Read the model definition and answer for the solid it produces. Units are mm, in the model's axes. Face numbers are marked on the shaded views. A direction names the side the tool comes from. Give positions to 0.01 mm unless a question says otherwise; leave off trailing zeros. Write each loop counter-clockwise with the first axis right and the second up, starting at its lowest first coordinate (ties: lowest second). Pieces come first, ordered by that corner, then holes. Notation, with made-up numbers: M -25,-20.5 L -7,-20.5 A32 cw -7,11.5 Z; hole C 87.5,0 d2. An arc over 180 degrees is marked long. Put each result on its own line as item: value.
from build123d import *

# Parameters (mm, degrees)
SKETCH1_W           = 84.03
SKETCH1_H           = 44.97
SKETCH1_W_2         = 0.71
SKETCH1_H_2         = 0.71
BOSS_EXTRUDE1_DEPTH = 4.61
CUT_EXTRUDE1_REACH  = 6.61
SKETCH2_R           = 1.25
SKETCH2_3_W         = 7.27
SKETCH2_3_H         = 4.6
CUT_EXTRUDE2_DEPTH  = 2.45
SKETCH2_4_R         = 6.72
SKETCH2_4_R_2       = 5.64
CUT_EXTRUDE3_DEPTH  = 1.75
SKETCH2_5_W         = 5.16
SKETCH2_5_H         = 14.14
SKETCH2_5_W_2       = 4.69
SKETCH2_5_H_2       = 2.4
SKETCH2_5_W_3       = 6.54
SKETCH2_5_H_3       = 7.3
SKETCH2_5_W_4       = 2.72
SKETCH2_5_H_4       = 6.27
CUT_EXTRUDE4_DEPTH  = 0.75


with BuildPart() as part:
    # Sketch1 → Boss-Extrude1 (new body)
    with BuildSketch(Plane(origin=(0, 0, 0), x_dir=(1, 0, 0), z_dir=(0, 1, 0))):
        with Locations((-42.015, -22.485)):
            Rectangle(SKETCH1_W, SKETCH1_H)
        with Locations((-74.615, -42.285)):
            Rectangle(SKETCH1_W_2, SKETCH1_H_2, mode=Mode.SUBTRACT)
        with Locations((-72.075, -42.285)):
            Rectangle(SKETCH1_W_2, SKETCH1_H_2, mode=Mode.SUBTRACT)
        with Locations((-69.535, -42.285)):
            Rectangle(SKETCH1_W_2, SKETCH1_H_2, mode=Mode.SUBTRACT)
        with Locations((-66.995, -42.285)):
            Rectangle(SKETCH1_W_2, SKETCH1_H_2, mode=Mode.SUBTRACT)
        with Locations((-64.455, -42.285)):
            Rectangle(SKETCH1_W_2, SKETCH1_H_2, mode=Mode.SUBTRACT)
        with Locations((-61.915, -42.285)):
            Rectangle(SKETCH1_W_2, SKETCH1_H_2, mode=Mode.SUBTRACT)
        with Locations((-59.375, -42.285)):
            Rectangle(SKETCH1_W_2, SKETCH1_H_2, mode=Mode.SUBTRACT)
        with Locations((-56.835, -42.285)):
            Rectangle(SKETCH1_W_2, SKETCH1_H_2, mode=Mode.SUBTRACT)
        with Locations((-54.295, -42.285)):
            Rectangle(SKETCH1_W_2, SKETCH1_H_2, mode=Mode.SUBTRACT)
        with Locations((-51.755, -42.285)):
            Rectangle(SKETCH1_W_2, SKETCH1_H_2, mode=Mode.SUBTRACT)
        with Locations((-49.215, -42.285)):
            Rectangle(SKETCH1_W_2, SKETCH1_H_2, mode=Mode.SUBTRACT)
        with Locations((-46.675, -42.285)):
            Rectangle(SKETCH1_W_2, SKETCH1_H_2, mode=Mode.SUBTRACT)
        with Locations((-44.135, -42.285)):
            Rectangle(SKETCH1_W_2, SKETCH1_H_2, mode=Mode.SUBTRACT)
        with Locations((-41.595, -42.285)):
            Rectangle(SKETCH1_W_2, SKETCH1_H_2, mode=Mode.SUBTRACT)
    extrude(amount=BOSS_EXTRUDE1_DEPTH)

    # Sketch2 → Cut-Extrude1 (cut, up to next)
    with BuildSketch(Plane(origin=(0, 4.61, 0), x_dir=(1, 0, 0), z_dir=(0, 1, 0)), mode=Mode.PRIVATE) as cut_extrude1_sk1:
        with Locations((-79.535, -4.45)):
            Circle(SKETCH2_R)
    cut_extrude1_tool1 = extrude(cut_extrude1_sk1.sketch, amount=-CUT_EXTRUDE1_REACH, mode=Mode.PRIVATE) & part.part
    add(cut_extrude1_tool1.solids().sort_by_distance((-79.535, 4.61, 4.45))[0], mode=Mode.SUBTRACT)
    # Sketch2 → Cut-Extrude1 (cut, up to next)
    with BuildSketch(Plane(origin=(0, 4.61, 0), x_dir=(1, 0, 0), z_dir=(0, 1, 0)), mode=Mode.PRIVATE) as cut_extrude1_sk2:
        with Locations((-4.5, -4.45)):
            Circle(SKETCH2_R)
    cut_extrude1_tool2 = extrude(cut_extrude1_sk2.sketch, amount=-CUT_EXTRUDE1_REACH, mode=Mode.PRIVATE) & part.part
    add(cut_extrude1_tool2.solids().sort_by_distance((-4.5, 4.61, 4.45))[0], mode=Mode.SUBTRACT)
    # Sketch2 → Cut-Extrude1 (cut, up to next)
    with BuildSketch(Plane(origin=(0, 4.61, 0), x_dir=(1, 0, 0), z_dir=(0, 1, 0)), mode=Mode.PRIVATE) as cut_extrude1_sk3:
        with Locations((-4.5, -35.3)):
            Circle(SKETCH2_R)
    cut_extrude1_tool3 = extrude(cut_extrude1_sk3.sketch, amount=-CUT_EXTRUDE1_REACH, mode=Mode.PRIVATE) & part.part
    add(cut_extrude1_tool3.solids().sort_by_distance((-4.5, 4.61, 35.3))[0], mode=Mode.SUBTRACT)
    # Sketch2 → Cut-Extrude1 (cut, up to next)
    with BuildSketch(Plane(origin=(0, 4.61, 0), x_dir=(1, 0, 0), z_dir=(0, 1, 0)), mode=Mode.PRIVATE) as cut_extrude1_sk4:
        with Locations((-79.535, -35.3)):
            Circle(SKETCH2_R)
    cut_extrude1_tool4 = extrude(cut_extrude1_sk4.sketch, amount=-CUT_EXTRUDE1_REACH, mode=Mode.PRIVATE) & part.part
    add(cut_extrude1_tool4.solids().sort_by_distance((-79.535, 4.61, 35.3))[0], mode=Mode.SUBTRACT)

    # Sketch2_3 → Cut-Extrude2 (cut)
    with BuildSketch(Plane(origin=(0, 4.61, 0), x_dir=(1, 0, 0), z_dir=(0, 1, 0))):
        with Locations((-70.605, -9.24)):
            Rectangle(SKETCH2_3_W, SKETCH2_3_H)
        with Locations((-42.515, -9.24)):
            Rectangle(SKETCH2_3_W, SKETCH2_3_H)
        with Locations((-13.355, -9.24)):
            Rectangle(SKETCH2_3_W, SKETCH2_3_H)
        with Locations((-13.355, -31.13)):
            Rectangle(SKETCH2_3_W, SKETCH2_3_H)
        with Locations((-42.515, -31.13)):
            Rectangle(SKETCH2_3_W, SKETCH2_3_H)
        with Locations((-70.605, -31.13)):
            Rectangle(SKETCH2_3_W, SKETCH2_3_H)
    extrude(amount=-CUT_EXTRUDE2_DEPTH, mode=Mode.SUBTRACT)

    # Sketch2_4 → Cut-Extrude3 (cut)
    with BuildSketch(Plane(origin=(0, 4.61, 0), x_dir=(1, 0, 0), z_dir=(0, 1, 0))):
        with Locations((-54.61, -20.79)):
            Circle(SKETCH2_4_R)
        with Locations((-29.26, -19.59)):
            Circle(SKETCH2_4_R_2)
    extrude(amount=-CUT_EXTRUDE3_DEPTH, mode=Mode.SUBTRACT)

    # Sketch2_5 → Cut-Extrude4 (cut)
    with BuildSketch(Plane(origin=(0, 4.61, 0), x_dir=(1, 0, 0), z_dir=(0, 1, 0))):
        with Locations((-72.86, -20.27)):
            Rectangle(SKETCH2_5_W, SKETCH2_5_H)
        with Locations((-64.665, -23.58)):
            Rectangle(SKETCH2_5_W_2, SKETCH2_5_H_2)
        with Locations((-22.14, -5.43)):
            Rectangle(SKETCH2_5_W_3, SKETCH2_5_H_3)
        with Locations((-3.35, -20.235)):
            Rectangle(SKETCH2_5_W_4, SKETCH2_5_H_4)
    extrude(amount=-CUT_EXTRUDE4_DEPTH, mode=Mode.SUBTRACT)


solid = part.part
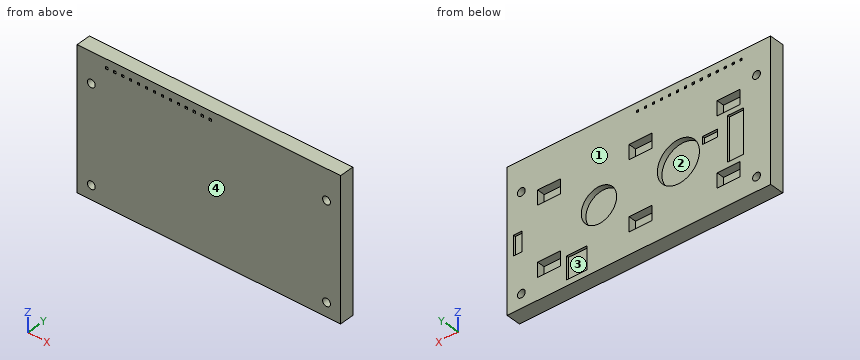
(1) Given pin 1 Ø1.4 at (x, z) = (-43.5, 32) entering from +Y, flat-ended and moving along its own axis, determine where the tip first touches the part or whether it passes through.
Result:
pin 1: stops at y = 2.16
(2) Which of the six approach directions +Z, -Z, +X, -X, +Y, -Y give full straight-line access (tool end or side, diameter ignored) to the marked faces 3 and 4?
Result:
face 3: +Y
face 4: +Z, -Z, +X, -X, -Y
(3) Straight lines are drawn through the part: line 1 along X through (y, z) = (1.05, 4.45) (3 decimals); line 2 along Z through (x, y) = (-42.5, 3.5); line 3 along Z through (x, y) = (-4.5, 2.65). For each, find the intervals that lie inside material, in ascending order. Write a range as from..to.
Result:
line 1: x = -84.03..-80.785, -78.285..-5.75, -3.25..0
line 2: z = 0..6.94, 11.54..28.83, 33.43..44.97
line 3: z = 0..3.2, 5.7..34.05, 36.55..44.97
(4) Section D-D on z = 19.59 is taken. Determine the outline of the cut face in (x, y), and give its area (3 significant figures).
Result:
outline: M -84.03,0 L 0,0 L 0,4.61 L -1.99,4.61 L -1.99,3.86 L -4.71,3.86 L -4.71,4.61 L -23.62,4.61 L -23.62,2.86 L -34.9,2.86 L -34.9,4.61 L -48,4.61 L -48,2.86 L -61.22,2.86 L -61.22,4.61 L -70.28,4.61 L -70.28,3.86 L -75.44,3.86 L -75.44,4.61 L -84.03,4.61 Z
area: 339 mm²
(5) Section C-C on z = 4.45 is taken. Determine the outline of the cut face in (x, y) (3 decimals), and give its area (3 significant figures).
Result:
outline: M -84.03,0 L -80.785,0 L -80.785,4.61 L -84.03,4.61 Z; M -78.285,0 L -5.75,0 L -5.75,4.61 L -18.87,4.61 L -18.87,3.86 L -25.41,3.86 L -25.41,4.61 L -78.285,4.61 Z; M -3.25,0 L 0,0 L 0,4.61 L -3.25,4.61 Z
area: 359 mm²
(6) For a pull along Z with two mould halves and no side action, classify the marked faces 1 and 2 as +Z half, -Z half, draft (parallel to the pull), parting line (faces both ways), or undercut.
Result:
face 1: draft
face 2: undercut
(7) Section B-B on x = -40 is taken. Determine the outline of the cut face in (y, z), and give its area (3 significant figures).
Result:
outline: M 0,0 L 4.61,0 L 4.61,6.94 L 2.16,6.94 L 2.16,11.54 L 4.61,11.54 L 4.61,28.83 L 2.16,28.83 L 2.16,33.43 L 4.61,33.43 L 4.61,44.97 L 0,44.97 Z
area: 185 mm²
(8) Section A-A on z = 35.3 is taken. Determine the outline of the cut face in (x, y) (3 decimals), and give its area (3 significant figures).
Result:
outline: M -84.03,0 L -80.785,0 L -80.785,4.61 L -84.03,4.61 Z; M -78.285,0 L -5.75,0 L -5.75,4.61 L -78.285,4.61 Z; M -3.25,0 L 0,0 L 0,4.61 L -3.25,4.61 Z
area: 364 mm²
